from build123d import *

# Parameters (mm, degrees)
F1_DEPTH = 16
F2_W     = 70
F2_H     = 3
F3_DEPTH = 2


with BuildPart() as f1:
    # F0 (on Front) → F1 (new body)
    with BuildSketch(Plane.XZ):
        with BuildLine():
            Line((94, 11), (0, 11))
            ThreePointArc((0, 11), (-11, 0), (0, -11))
            Line((0, -11), (19, -11))
            ThreePointArc((19, -11), (21.768112, -11.836161), (23.61039, -14.064979))
            ThreePointArc((23.61039, -14.064979), (52.373093, -47.586467), (95.296574, -58.00559))
            ThreePointArc((95.296574, -58.00559), (101.981922, -58.918984), (107.67752, -62.536763))
            Line((107.67752, -62.536763), (108.967018, -61))
            ThreePointArc((108.967018, -61), (102.665945, -57.039589), (95.296574, -56))
            ThreePointArc((95.296574, -56), (53.4812, -45.919824), (25.454545, -13.29097))
            ThreePointArc((25.454545, -13.29097), (22.875357, -10.170626), (19, -9))
            Line((19, -9), (0, -9))
            ThreePointArc((0, -9), (-9, 0), (0, 9))
            Line((0, 9), (94, 9))
            Line((94, 9), (94, 11))
        make_face()
    extrude(amount=-F1_DEPTH)

    # F2 (on face) → F3 (join)
    with BuildSketch(Plane.XY.offset(11)):
        with Locations((59, -1.5)):
            Rectangle(F2_W, F2_H)
    extrude(amount=-F3_DEPTH)


solid = f1.part
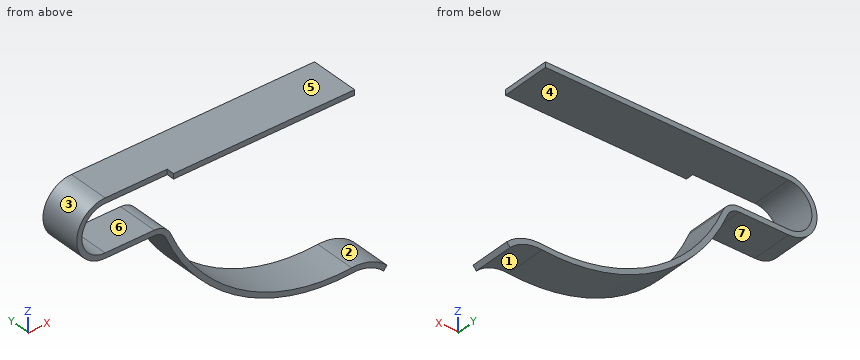
Can you work these out from the model? Positions are in its coordinate system, mm. Face numbers are marked on the shaded views. A direction names the side the tool comes from. Give positions to 0.01 mm unless a question says otherwise; leave off trailing zeros. Order: outer loops, then holes, each group sorted by start corner. A loop starts at its lowest first (then second) coordinate and runs counter-clockwise, first axis right, second up. Notation, with made-up numbers: M 55,61 L 113,61 A15 ccw 113,72 Z; hole C 41.5,-7 d6. An arc over 180 degrees is marked long. One line per item, written item: value.
Item 1: If we section it at C-C on y = 6: Write out the boundary of the cut face in (x, z).
Verdict:
outline: M 0,-11 L 19,-11 A5 cw 23.61,-14.06 A72 ccw 95.3,-58.01 A15.81 cw 107.68,-62.54 L 108.97,-61 A17.81 ccw 95.3,-56 A70 cw 25.45,-13.29 A7 ccw 19,-9 L 0,-9 A9 cw 0,9 L 94,9 L 94,11 L 0,11 A11 ccw Z
Item 2: If we section it at B-B on z = 0: Write out the boundary of the cut face in (x, y), and give its area (3 significant figures).
Verdict:
outline: M -11,0 L -9,0 L -9,16 L -11,16 Z
area: 32.0 mm2
Item 3: If we section it at D-D on x = 70: Write out the boundary of the cut face in (y, z), and give its area (3 significant figures).
Verdict:
outline: M -3,9 L 16,9 L 16,11 L -3,11 Z; M 0,-55.37 L 16,-55.37 L 16,-53.28 L 0,-53.28 Z
area: 71.4 mm2
Item 4: If we mould it in two halves opening along Z, with no side actions, what happens to the marked faces 1, 2, 3 and 4? For each: pulls with the +Z half, pulls with the -Z half, needs draft (parallel to the pull), parting line crosses it, or undercut.
Verdict:
face 1: pulls with the -Z half
face 2: pulls with the +Z half
face 3: parting line crosses it
face 4: undercut
Item 5: Please list where these lines run through material, in increasing order: line 1 (Z direction, x = 1, y = 3); line 2 (Z direction, x = 39, y = -0.75); line 3 (Z direction, x = 54.5, y = 4.5).
Verdict:
line 1: -11 to -9, 9 to 11
line 2: 9 to 11
line 3: -48.84 to -46.53, 9 to 11
Item 6: If we section it at A-A on x = 50: Write out the boundary of the cut face in (y, z), and give its area (3 significant figures).
Verdict:
outline: M -3,9 L 16,9 L 16,11 L -3,11 Z; M 0,-46.07 L 16,-46.07 L 16,-43.65 L 0,-43.65 Z
area: 76.7 mm2
Item 7: For pin 1 (22 mm diameter, centred on x = 68, z = -41, fed in from -Y); pin 2 (0.6 mm diameter, centred on y = -1, z = 10, fed in from -X); pin 3 (2 mm diameter, centred on y = 4.5, z = 9.5, fed in from +X), each with a flat end and sliding along its axis, tell me the tip position at first contact or that it passes through.
Verdict:
pin 1: y = 0
pin 2: x = 24
pin 3: x = 94
Item 8: For the marked faces 5, 6 and 7, which set-ups out of +Z, -Z, +X, -X, +Y, -Y let a thin tool reach every point of the face, with its end or its side?
Verdict:
face 5: +Z, +X, -X, +Y, -Y
face 6: +X, +Y, -Y
face 7: -Z, -X, +Y, -Y
